Geometry check sheet. Reference: the model listing, model coordinates, mm. Face numbers are marked on the shaded views. A direction names the side the tool comes from. Round coordinates to 2 decimals unless told otherwise and drop trailing zeros. Order: outer loops, then holes, each group sorted by start corner. A loop starts at its lowest first (then second) coordinate and runs counter-clockwise, first axis right, second up. Notation, with made-up numbers: (51, 31.25) - (71, 31.25) arc R19 cw to (71, 65.25) - close; hole circle Ø5 at (72, 44.25). An arc over 180 degrees is marked (long way). Write each question's results on one line, items separated by ' | '.
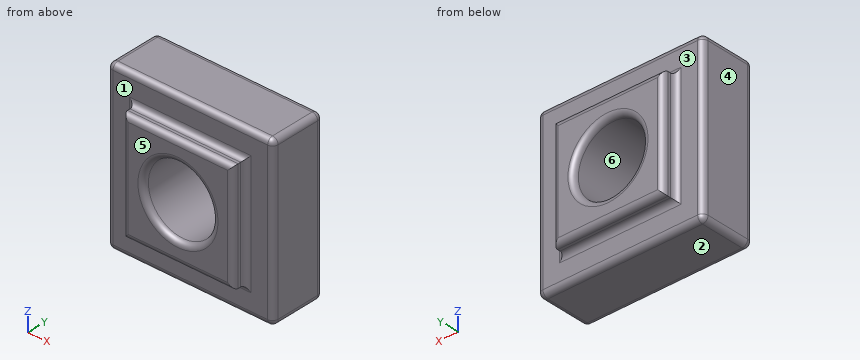
```python
from build123d import *

# Parameters (mm, degrees)
F0_W     = 101.6
F0_H     = 101.6
F0_R     = 31.75
F1_DEPTH = 38.1
F0_W_2   = 152.4
F0_H_2   = 152.4
F2_DEPTH = 25.4
F3_R     = 5.08


with BuildPart() as f1:
    # F0 (on Front) → F1 (new body, symmetric)
    with BuildSketch(Plane.XZ):
        Rectangle(F0_W, F0_H)
        Circle(F0_R, mode=Mode.SUBTRACT)
    extrude(amount=F1_DEPTH, both=True)

    # F0 (on Front) → F2 (join, symmetric)
    with BuildSketch(Plane.XZ):
        Rectangle(F0_W_2, F0_H_2)
        Rectangle(F0_W, F0_H, mode=Mode.SUBTRACT)
    extrude(amount=F2_DEPTH, both=True)

    # F3
    f3_edges = [f1.edges().sort_by_distance(p)[0] for p in [
        (76.2, 25.4, 0),
        (0, 25.4, 76.2),
        (-76.2, 25.4, 0),
        (0, 25.4, -76.2),
        (0, 25.4, 50.8),
        (50.8, 25.4, 0),
        (0, 25.4, -50.8),
        (-50.8, 25.4, 0),
        (50.8, 38.1, 0),
        (0, 38.1, 50.8),
        (-50.8, 38.1, 0),
        (0, 38.1, -50.8),
        (-31.75, 38.1, 0),
        (50.8, -38.1, 0),
        (0, -38.1, 50.8),
        (-50.8, -38.1, 0),
        (0, -38.1, -50.8),
        (-31.75, -38.1, 0),
        (76.2, -25.4, 0),
        (0, -25.4, 76.2),
        (-76.2, -25.4, 0),
        (0, -25.4, -76.2),
        (0, -25.4, 50.8),
        (50.8, -25.4, 0),
        (0, -25.4, -50.8),
        (-50.8, -25.4, 0),
        (76.2, 0, -76.2),
        (-76.2, 0, -76.2),
        (76.2, 0, 76.2),
        (-76.2, 0, 76.2),
    ]]
    fillet(f3_edges, radius=F3_R)


solid = f1.part
```
(1) Section check D-D (z = 40.5). Record the cut outline in (x, y).
Answers follow:
outline: (-76.2, -20.32) arc R5.08 ccw to (-71.12, -25.4) - (-55.88, -25.4) arc R5.08 cw to (-50.8, -30.48) - (-50.8, -33.02) arc R5.08 ccw to (-45.72, -38.1) - (45.72, -38.1) arc R5.08 ccw to (50.8, -33.02) - (50.8, -30.48) arc R5.08 cw to (55.88, -25.4) - (71.12, -25.4) arc R5.08 ccw to (76.2, -20.32) - (76.2, 20.32) arc R5.08 ccw to (71.12, 25.4) - (55.88, 25.4) arc R5.08 cw to (50.8, 30.48) - (50.8, 33.02) arc R5.08 ccw to (45.72, 38.1) - (-45.72, 38.1) arc R5.08 ccw to (-50.8, 33.02) - (-50.8, 30.48) arc R5.08 cw to (-55.88, 25.4) - (-71.12, 25.4) arc R5.08 ccw to (-76.2, 20.32) - close
(2) Material ranges on line 1 (Z direction, x = 0, y = 2.5); line 2 (Z direction, x = -21, y = 2.5); line 3 (Y direction, x = -65, z = 16.5), recorded low to high.
Answers follow:
line 1: -76.2 to -31.75, 31.75 to 76.2 | line 2: -76.2 to -23.81, 23.81 to 76.2 | line 3: -25.4 to 25.4
(3) Depth check by flat-ended pin: pin 1 Ø3 at (x, y) = (16.5, -32) entering from -Z; pin 2 Ø4 at (x, z) = (-12, 32) entering from +Y; pin 3 Ø2 at (y, z) = (32.5, -15.5) entering from -X. Enter the tip coordinate at first touch or a pass-through.
Answers follow:
pin 1: z = -50.8 | pin 2: y = 38.06 | pin 3: x = -50.8
(4) Draft check along X on the marked faces 4, 5 and 6. Enter one of: released by +X, released by -X, zero draft, split by the parting line, or undercut.
Answers follow:
face 4: released by -X | face 5: zero draft | face 6: undercut
(5) Section check C-C (y = 14). Record the cut outline in (x, z).
Answers follow:
outline: (-76.2, -71.12) arc R5.08 ccw to (-71.12, -76.2) - (71.12, -76.2) arc R5.08 ccw to (76.2, -71.12) - (76.2, 71.12) arc R5.08 ccw to (71.12, 76.2) - (-71.12, 76.2) arc R5.08 ccw to (-76.2, 71.12) - close; hole circle Ø63.5 at (0, 0)
(6) Access from +Z, -Z, +X, -X, +Y, -Y to the whole of each face (thin tool, end or side, straight path). Record for the marked faces 1, 2 and 3.
Answers follow:
face 1: -Y | face 2: -Z, +X, -X, +Y, -Y | face 3: +Y
